from build123d import *

# Parameters (mm, degrees)
BOSS_EXTRUDE1_DEPTH               = 450
RIGHTSIDEHOLES_SKETCH3_R          = 1.5875
RIGHTSIDEHOLES_CUT_EXTRUDE1_DEPTH = 3.175
FRONTSIDEHOLES_SKETCH4_R          = 1.5875
FRONTSIDEHOLES_CUT_EXTRUDE2_DEPTH = 3.175


with BuildPart() as part:
    # Sketch2 → Boss-Extrude1 (new body)
    with BuildSketch(Plane(origin=(0, 0, 0), x_dir=(1, 0, 0), z_dir=(0, 1, 0))):
        Polygon((0, 31.75), (3.175, 31.75), (3.175, 3.175), (31.75, 3.175), (31.75, 0), (0, 0), align=None)
    extrude(amount=BOSS_EXTRUDE1_DEPTH)

    # RightSideHoles-Sketch3 → RightSideHoles-Cut-Extrude1 (cut)
    with BuildSketch(Plane.XY):
        with Locations((14.2875, 81.1125)):
            Circle(RIGHTSIDEHOLES_SKETCH3_R)
        with Locations((23.8125, 81.1125)):
            Circle(RIGHTSIDEHOLES_SKETCH3_R)
        with Locations((14.2875, 87.4625)):
            Circle(RIGHTSIDEHOLES_SKETCH3_R)
        with Locations((23.8125, 87.4625)):
            Circle(RIGHTSIDEHOLES_SKETCH3_R)
        with Locations((14.2875, 438.8875)):
            Circle(RIGHTSIDEHOLES_SKETCH3_R)
        with Locations((14.2875, 426.1875)):
            Circle(RIGHTSIDEHOLES_SKETCH3_R)
        with Locations((23.8125, 438.8875)):
            Circle(RIGHTSIDEHOLES_SKETCH3_R)
        with Locations((23.8125, 426.1875)):
            Circle(RIGHTSIDEHOLES_SKETCH3_R)
        with Locations((14.2875, 332.602644)):
            Circle(RIGHTSIDEHOLES_SKETCH3_R)
        with Locations((23.8125, 332.602644)):
            Circle(RIGHTSIDEHOLES_SKETCH3_R)
        with Locations((14.2875, 319.902644)):
            Circle(RIGHTSIDEHOLES_SKETCH3_R)
        with Locations((23.8125, 319.902644)):
            Circle(RIGHTSIDEHOLES_SKETCH3_R)
        with Locations((14.2875, 7.9375)):
            Circle(RIGHTSIDEHOLES_SKETCH3_R)
        with Locations((23.8125, 7.9375)):
            Circle(RIGHTSIDEHOLES_SKETCH3_R)
        with Locations((14.2875, 165)):
            Circle(RIGHTSIDEHOLES_SKETCH3_R)
        with Locations((14.2875, 260)):
            Circle(RIGHTSIDEHOLES_SKETCH3_R)
        with Locations((14.2875, 355)):
            Circle(RIGHTSIDEHOLES_SKETCH3_R)
    extrude(amount=-RIGHTSIDEHOLES_CUT_EXTRUDE1_DEPTH, mode=Mode.SUBTRACT)

    # FrontSideHoles-Sketch4 → FrontSideHoles-Cut-Extrude2 (cut)
    with BuildSketch(Plane.ZY):
        with Locations((-23.8125, 81.1125)):
            Circle(FRONTSIDEHOLES_SKETCH4_R)
        with Locations((-14.2875, 81.1125)):
            Circle(FRONTSIDEHOLES_SKETCH4_R)
        with Locations((-23.8125, 87.4625)):
            Circle(FRONTSIDEHOLES_SKETCH4_R)
        with Locations((-14.2875, 87.4625)):
            Circle(FRONTSIDEHOLES_SKETCH4_R)
        with Locations((-23.8125, 438.8875)):
            Circle(FRONTSIDEHOLES_SKETCH4_R)
        with Locations((-14.2875, 438.8875)):
            Circle(FRONTSIDEHOLES_SKETCH4_R)
        with Locations((-23.8125, 426.1875)):
            Circle(FRONTSIDEHOLES_SKETCH4_R)
        with Locations((-14.2875, 426.1875)):
            Circle(FRONTSIDEHOLES_SKETCH4_R)
        with Locations((-14.2875, 338.177644)):
            Circle(FRONTSIDEHOLES_SKETCH4_R)
        with Locations((-14.2875, 319.652644)):
            Circle(FRONTSIDEHOLES_SKETCH4_R)
        with Locations((-14.2875, 165)):
            Circle(FRONTSIDEHOLES_SKETCH4_R)
        with Locations((-14.2875, 260)):
            Circle(FRONTSIDEHOLES_SKETCH4_R)
        with Locations((-14.2875, 355)):
            Circle(FRONTSIDEHOLES_SKETCH4_R)
    extrude(amount=-FRONTSIDEHOLES_CUT_EXTRUDE2_DEPTH, mode=Mode.SUBTRACT)


solid = part.part
Part model, mm, in its own coordinate system. A direction names the side the tool comes from. Give positions to 0.01 mm unless a question says otherwise; leave off trailing zeros. Write each loop counter-clockwise with the first axis right and the second up, starting at its lowest first coordinate (ties: lowest second). Pieces come first, ordered by that corner, then holes.
1) Which spindle directions (+Z, -Z, +X, -X, +Y, -Y) get a long thin tool onto all of the face, cutting with end or side? Do faces 1 (the face through (17, 222, -3.175)), 2 (the face through (9, 0, -3)). Say none if no direction does.
Resolved:
face 1: -Z, +X, +Y, -Y
face 2: +Z, -Z, +X, -X, -Y
2) Pin check, flat tips, straight feed: pin 1 (3.5 mm diameter, centred on x = 23.81, y = 332.6, fed in from -Z) (3 decimals); pin 2 (12 mm diameter, centred on y = 184.5, z = -21, fed in from -X); pin 3 (2.5 mm diameter, centred on y = 87.46, z = -14.29, fed in from +X); pin 4 (5 mm diameter, centred on y = 350, z = -9.5, fed in from +X) (3 decimals). Stop position of each tip, or through.
Resolved:
pin 1: stops at z = -3.175
pin 2: stops at x = 0
pin 3: passes through
pin 4: stops at x = 3.175
3) Cut at A-A on y = 395. Write the cut outline in (x, z) (3 decimals), then the cut area to 3 significant figures.
Resolved:
outline: (0, -31.75) - (3.175, -31.75) - (3.175, -3.175) - (31.75, -3.175) - (31.75, 0) - (0, 0) - close
area: 192 mm2
4) Probe L1, parallel to Y at x = 2.5, z = -23.5; L2, parallel to X at y = 260, z = -1.8 (3 decimals); L3, parallel to X at y = 206.5, z = -29 (3 decimals). List the from-to ranges inside material, lowest first.
Resolved:
L1: y = 0 to 79.56, 82.67 to 85.91, 89.02 to 424.63, 427.74 to 437.33, 440.44 to 450
L2: x = 0 to 12.7, 15.875 to 31.75
L3: x = 0 to 3.175
5) Cut at B-B on x = 9. Write the cut outline in (y, z) (3 decimals), then the cut area to 3 significant figures.
Resolved:
outline: (0, -3.175) - (450, -3.175) - (450, 0) - (0, 0) - close
area: 1,430 mm2
